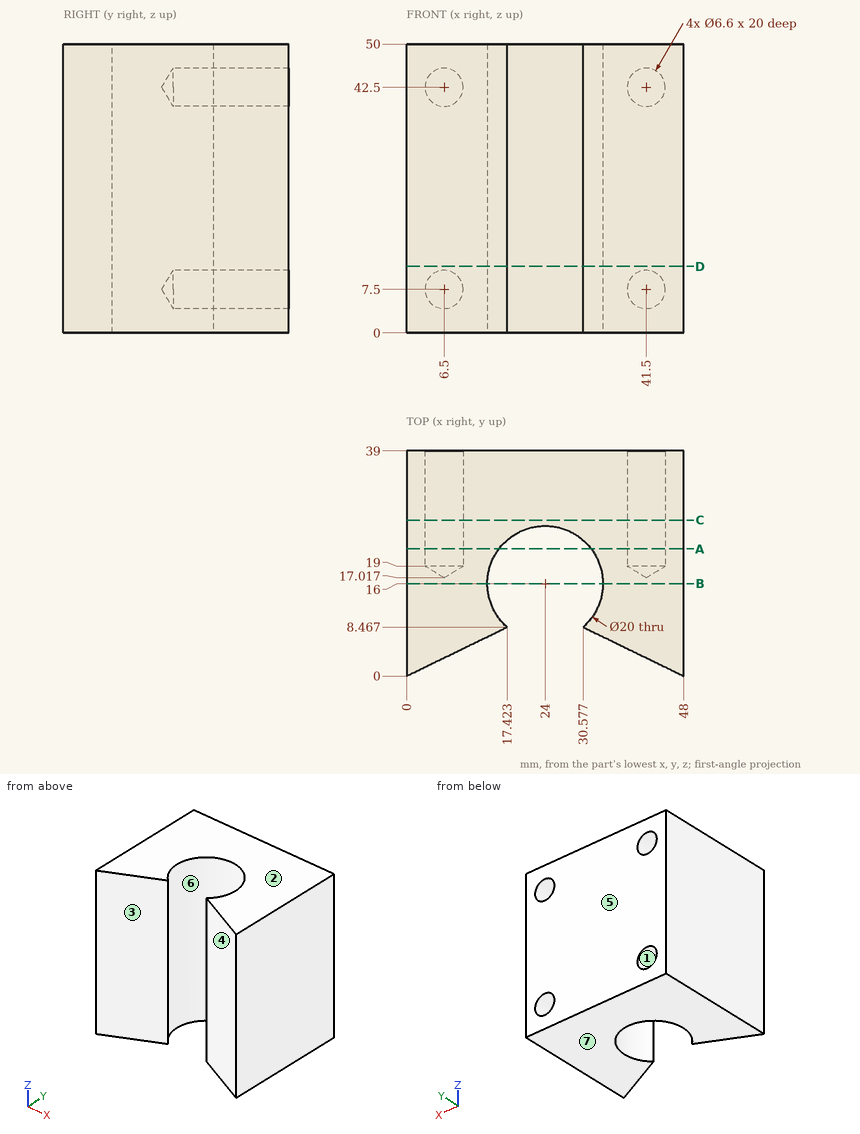
Answer from the drawing. Dimensions are ordinates in mm from the lowest x, y and z of the part. A direction names the side the tool comes from. Coordinates: 2 decimals unless noted, no trailing zeros. Loops run counter-clockwise (first coordinate to the right, second up) from the corner with the lowest first, then second, coordinate; pieces in that order, holes last.
1) Flat-ended cylindrical pins translate along their axes: pin 1 (10.5 mm diameter, centred on x = 41.5, z = 7.5, fed in from -Y); pin 2 (2 mm diameter, centred on x = 35, z = 44.5, fed in from -Y); pin 3 (5.5 mm diameter, centred on x = 6.5, z = 42.5, fed in from +Y). Find the tip coordinate at first contact, or state that the pin passes through.
Results:
pin 1: stops at y = 0.61
pin 2: stops at y = 5.83
pin 3: stops at y = 18.67
2) Section C-C (y = 27) is taken. Give the vertices of the cut face in (x, z), plus the area to 3 significant figures.
Results:
outline: (0, 0) - (48, 0) - (48, 50) - (0, 50) - close; hole circle Ø6.6 at (6.5, 7.5); hole circle Ø6.6 at (6.5, 42.5); hole circle Ø6.6 at (41.5, 7.5); hole circle Ø6.6 at (41.5, 42.5)
area: 2,260 mm2
3) Section A-A (y = 22) is taken. Give the vertices of the cut face in (x, z).
Results:
outline: (0, 0) - (16, 0) - (16, 50) - (0, 50) - close; (32, 0) - (48, 0) - (48, 50) - (32, 50) - close; hole circle Ø6.6 at (6.5, 7.5); hole circle Ø6.6 at (6.5, 42.5); hole circle Ø6.6 at (41.5, 7.5); hole circle Ø6.6 at (41.5, 42.5)
4) Section B-B (y = 16) is taken. Give the vertices of the cut face in (x, z).
Results:
outline: (0, 0) - (14, 0) - (14, 50) - (0, 50) - close; (34, 0) - (48, 0) - (48, 50) - (34, 50) - close
5) For a pull along Y with two mould halves and no side action, classify the marked faces 4, 5, 6 and 7 as +Y half, -Y half, draft (parallel to the pull), parting line (faces both ways), or undercut.
Results:
face 4: -Y half
face 5: +Y half
face 6: undercut
face 7: draft
6) Section D-D (z = 11.5) is taken. Give the vertices of the cut face in (x, y), plus the area to 3 significant figures.
Results:
outline: (0, 0) - (17.42, 8.47) arc R10 cw (long way) to (30.58, 8.47) - (48, 0) - (48, 39) - (0, 39) - close
area: 1,320 mm2
7) For the marked faces 1, 2 and 3, determine the directions among +Z, -Z, +X, -X, +Y, -Y from which every point of the face is accessible in a straight line to the end or side of a thin tool.
Results:
face 1: +Y
face 2: +Z, +X, -X, +Y, -Y
face 3: +Z, -Z, -Y
8) Consider probe 1 along Z at (x, y) = (6.5, 30.5); probe 2 along X at (y, z) = (34, 7.5); probe 3 along X at (y, z) = (16, 27). Determine where each line is inside the solid, lowest interval first.
Results:
probe 1: z = 0 to 4.2, 10.8 to 39.2, 45.8 to 50
probe 2: x = 0 to 3.2, 9.8 to 38.2, 44.8 to 48
probe 3: x = 0 to 14, 34 to 48
